Model file for the job. Use its own axes, mm. Coordinates: 2 decimals unless noted, no trailing zeros. Order: outer loops, then holes, each group sorted by start corner. A loop starts at its lowest first (then second) coordinate and runs counter-clockwise, first axis right, second up.
Autodesk Inventor part; units mm, degrees
ref_plane "YZ Plane" through (0, 0, 0) normal (1, 0, 0) x (0, 1, 0)
ref_plane "XZ Plane" through (0, 0, 0) normal (0, 1, 0) x (-1, 0, 0)
ref_plane "XY Plane" through (0, 0, 0) normal (0, 0, 1) x (1, 0, 0)
sketch "Sketch1" plane through (0, 0, 0) normal (0, 0, 1) x (1, 0, 0)
  line L0 (0, 0) -> (2.95, 0)
  line L1 (2.95, 0) -> (2.95, 9.5)
  line L2 (0, 0) -> (0, 10.5)
  line L3 (0, 10.5) -> (4.5, 10.5)
  line L4 (4.5, 10.5) -> (4.5, 9.5)
  line L5 (4.5, 9.5) -> (2.95, 9.5)
  dimension "d0" = 2.95
  dimension "d1" = 9.5
  dimension "d2" = 10.5
  dimension "d3" = 4.5
revolve "Revolution1" add sketch "Sketch1" angle 360 about axis through (0, 0, 0) along (0, 1, 0)
sketch "Sketch2" plane through (0, 10.5, 0) normal (0, 1, 0) x (1, 0, 0)
  point P0 (0, 0)
  point P1 (0, 0)
hole "Hole1" at (0, 10.5, 0) direction (0, -1, 0) diameter 3.242 end through all
fillet "Fillet1" radius 1 1 edges at (-2.95, 0, 0)
properties part number "M4 Rivet nut" material "Brass, Soft Yellow, Welded"
Q1. Drop flat-ended pins along their axis: P1, Ø1, axis at x = -3, z = -0.5, coming from the -Y side; P2, Ø1.5, axis at y = 3.5, z = 0.5, coming from the +X side; P3, Ø5, axis at x = -2.5, y = 8, coming from the +Z side. Give the stop position or say it passes through.
Established:
P1: stops at y = 0.19
P2: stops at x = 2.95
P3: stops at z = 4.47
Q2. Cut at C-C, the plane y = 6.25. List the corners of the cut face in (x, z).
Established:
outline: circle Ø5.9 at (0, 0); hole circle Ø3.24 at (0, 0)
Q3. Cut at A-A, the plane z = 0. List the corners of the cut face in (x, y).
Established:
outline: (-4.5, 9.5) - (-2.95, 9.5) - (-2.95, 1) arc R1 ccw to (-1.95, 0) - (-1.62, 0) - (-1.62, 10.5) - (-4.5, 10.5) - close; (1.62, 0) - (1.95, 0) arc R1 ccw to (2.95, 1) - (2.95, 9.5) - (4.5, 9.5) - (4.5, 10.5) - (1.62, 10.5) - close
Q4. Probe line 1 (X direction, y = 5, z = 0); line 2 (Y direction, x = -2, z = -2.75). List the from-to ranges inside material, lowest first.
Established:
line 1: x = -2.95 to -1.62, 1.62 to 2.95
line 2: y = 9.5 to 10.5
Q5. Cut at D-D, the plane x = 3.75. List the corners of the cut face in (y, z), plus the area to 3 significant figures.
Established:
outline: (9.5, -2.49) - (10.5, -2.49) - (10.5, 2.49) - (9.5, 2.49) - close
area: 4.97 mm2
Q6. Cut at B-B, the plane x = 0. List the corners of the cut face in (y, z), plus the area to 3 significant figures.
Established:
outline: (0, -1.95) arc R1 ccw to (1, -2.95) - (9.5, -2.95) - (9.5, -4.5) - (10.5, -4.5) - (10.5, -1.62) - (0, -1.62) - close; (0, 1.62) - (10.5, 1.62) - (10.5, 4.5) - (9.5, 4.5) - (9.5, 2.95) - (1, 2.95) arc R1 ccw to (0, 1.95) - close
area: 30.6 mm2
Q7. Mould opens along Z. For faces 1 (the face through (1, 9.5, 3)), 2 (the face through (1.438, 5.176, 0.748)), 3 (the face through (-2.947, 5.31, -0.13)) say: pulls with the +Z half, pulls with the -Z half, needs draft (parallel to the pull), parting line crosses it, or undercut.
Established:
face 1: needs draft
face 2: undercut
face 3: parting line crosses it
